The listing builds one solid part. Answer for the finished solid, in the listing's coordinates (mm). A direction names the side the tool comes from. Round coordinates to 2 decimals unless told otherwise and drop trailing zeros. Loops run counter-clockwise (first coordinate to the right, second up) from the corner with the lowest first, then second, coordinate; pieces in that order, holes last. Notation, with made-up numbers: (-23.5, 10) - (-13.5, 10) arc R6 cw to (-13.5, 18) - close; hole circle Ø9 at (7.5, -24.5). An arc over 180 degrees is marked (long way). One line per item, written item: value.
```python
from build123d import *

# Parameters (mm, degrees)
F0_W     = 10.517747
F0_H     = 12.7
F1_DEPTH = 6.35


with BuildPart() as f1:
    # F0 (on Top) → F1 (new body)
    with BuildSketch(Plane.XY):
        with Locations((-6.54676, 6.35)):
            Rectangle(F0_W, F0_H)
        Polygon((-1.287887, 12.7), (-1.287887, 0), (-1.287887, -5.08), (6.332113, -5.08), (6.332113, 2.54), (3.792113, 2.54), (3.792113, 10.16), (6.332113, 10.16), (6.332113, 17.78), (-1.287887, 17.78), align=None)
    extrude(amount=F1_DEPTH)


solid = f1.part
```
1) For a pull along Y with two mould halves and no side action, classify faces 4 (the flat face through (-7, 0, 3)), 5 (the flat face through (3.792, 6, 3)), 6 (the flat face through (-7, 12.7, 3)) as released by +Y, released by -Y, zero draft, split by the parting line, or undercut.
Final values:
face 4: released by -Y
face 5: undercut
face 6: released by +Y
2) A cutting plane is placed at B-B on z = 3. Give the vertices of the cut face in (x, y).
Final values:
outline: (-11.81, 0) - (-1.29, 0) - (-1.29, -5.08) - (6.33, -5.08) - (6.33, 2.54) - (3.79, 2.54) - (3.79, 10.16) - (6.33, 10.16) - (6.33, 17.78) - (-1.29, 17.78) - (-1.29, 12.7) - (-11.81, 12.7) - close
3) Each of these flat-tipped pins is pushed along its axis until it touches: pin 1 Ø3 at (x, z) = (-8.5, 4) entering from -Y; pin 2 Ø1 at (y, z) = (6.5, 3) entering from +X. Where does it stop, or does it pass through?
Final values:
pin 1: y = 0
pin 2: x = 3.79
4) Consider L1, parallel to Y at x = 4.25, z = 1.75; L2, parallel to X at y = 16.25, z = 4.75; L3, parallel to Y at x = -8, z = 3.75. Determine where each line is inside the solid, lowest interval first.
Final values:
L1: -5.08 to 2.54, 10.16 to 17.78
L2: -1.29 to 6.33
L3: 0 to 12.7
5) A cutting plane is placed at A-A on x = 5. Give the vertices of the cut face in (y, z), and give its area (3 significant figures).
Final values:
outline: (-5.08, 0) - (2.54, 0) - (2.54, 6.35) - (-5.08, 6.35) - close; (10.16, 0) - (17.78, 0) - (17.78, 6.35) - (10.16, 6.35) - close
area: 96.8 mm2
6) A cutting plane is placed at C-C on x = -10.25. Give the vertices of the cut face in (y, z), and give its area (3 significant figures).
Final values:
outline: (0, 0) - (12.7, 0) - (12.7, 6.35) - (0, 6.35) - close
area: 80.6 mm2
7) For faces 1 (the flat face through (-1.288, 15, 3)), 2 (the flat face through (5, 10.16, 3)), 3 (the flat face through (-1.288, -3, 3)), determine the directions among +Z, -Z, +X, -X, +Y, -Y from which every point of the face is accessible in a straight line to the end or side of a thin tool.
Final values:
face 1: +Z, -Z, -X, +Y
face 2: +Z, -Z, +X
face 3: +Z, -Z, -X, -Y
8) A cutting plane is placed at D-D on y = 15.25. Give the vertices of the cut face in (x, z).
Final values:
outline: (-1.29, 0) - (6.33, 0) - (6.33, 6.35) - (-1.29, 6.35) - close
